Source: three-view drawing plus pictorial views. Frame: mm from the lowest corner of the part. A direction names the side the tool comes from. Coordinates: 2 decimals unless noted, no trailing zeros. Order: outer loops, then holes, each group sorted by start corner. A loop starts at its lowest first (then second) coordinate and runs counter-clockwise, first axis right, second up. Notation, with made-up numbers: M -14.5,86.25 L -3.5,86.25 A31 cw -3.5,123.25 Z; hole C -1,-7.5 d7. An arc over 180 degrees is marked long. One line per question, with ' | ' between items.
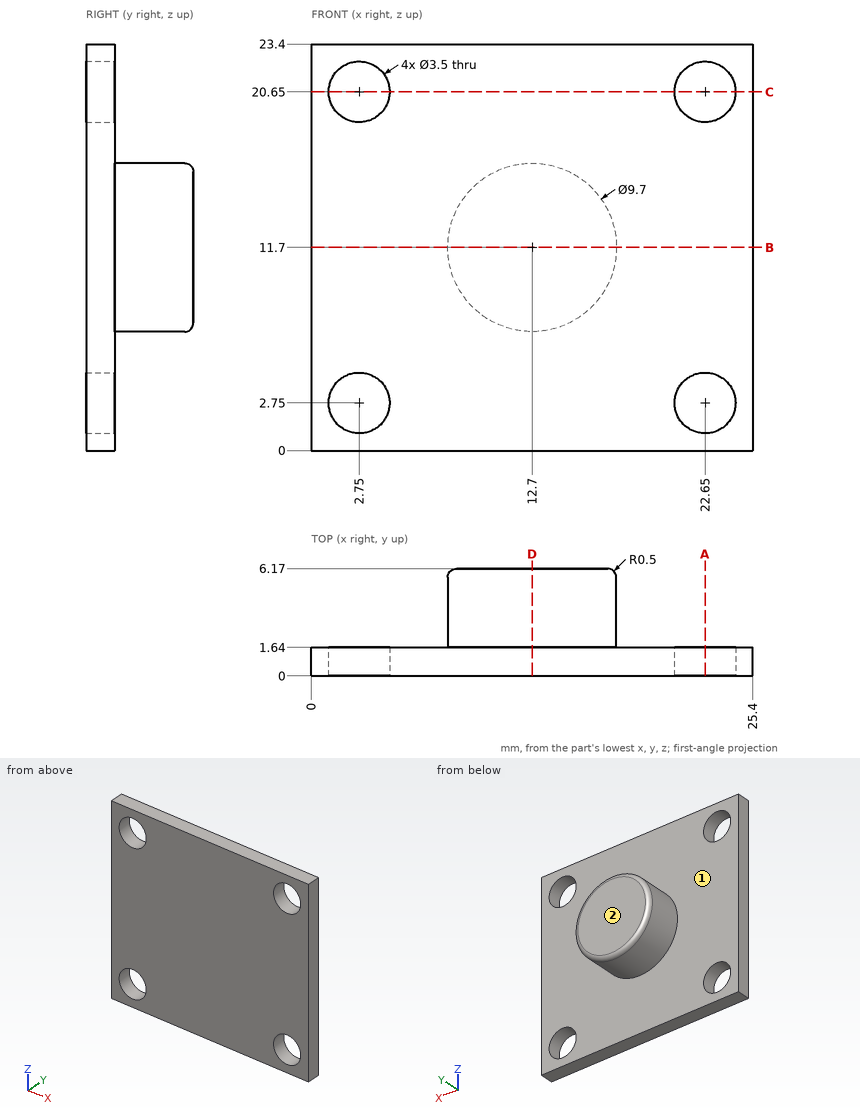
1. Section C-C, the plane z = 20.65. Output: boundary loops of the cut face in (x, y).
Response values:
outline: M 0,0 L 1,0 L 1,1.64 L 0,1.64 Z; M 4.5,0 L 20.9,0 L 20.9,1.64 L 4.5,1.64 Z; M 24.4,0 L 25.4,0 L 25.4,1.64 L 24.4,1.64 Z
2. Section D-D, the plane x = 12.7. Output: boundary loops of the cut face in (y, z), and give its area (3 significant figures).
Response values:
outline: M 0,0 L 1.64,0 L 1.64,6.85 L 5.67,6.85 A0.5 ccw 6.17,7.35 L 6.17,16.05 A0.5 ccw 5.67,16.55 L 1.64,16.55 L 1.64,23.4 L 0,23.4 Z | area: 82.2 mm^2
3. Access query for the marked faces 1 and 2. Directions: +Z, -Z, +X, -X, +Y, -Y. A direction counts if a zero-diameter tool reaches every point of the face in a straight line with its end or side. Return the directions, or none.
Response values:
face 1: +Y | face 2: +Z, -Z, +X, -X, +Y
4. Pin query (flat end, axial travel): P1, Ø5.5, axis at x = 2.75, z = 2.75, coming from the +Y side; P2, Ø1, axis at y = 4, z = 8, coming from the -X side. Return the tip coordinate at first contact, or that it passes through.
Response values:
P1: stops at y = 1.64 | P2: stops at x = 9.06
5. Section A-A, the plane x = 22.65. Output: boundary loops of the cut face in (y, z), and give its area (3 significant figures).
Response values:
outline: M 0,0 L 1.64,0 L 1.64,1 L 0,1 Z; M 0,4.5 L 1.64,4.5 L 1.64,18.9 L 0,18.9 Z; M 0,22.4 L 1.64,22.4 L 1.64,23.4 L 0,23.4 Z | area: 26.9 mm^2
6. Material intervals for line 1 (X direction, y = 1.35, z = 20.65); line 2 (Z direction, x = 22.65, y = 0.7); line 3 (Y direction, x = 6, z = 2.75), sorted ascending. Write a range as [from, to].
Response values:
line 1: x = [0, 1], [4.5, 20.9], [24.4, 25.4] | line 2: z = [0, 1], [4.5, 18.9], [22.4, 23.4] | line 3: y = [0, 1.64]
7. Section B-B, the plane z = 11.7. Output: boundary loops of the cut face in (x, y).
Response values:
outline: M 0,0 L 25.4,0 L 25.4,1.64 L 17.55,1.64 L 17.55,5.67 A0.5 ccw 17.05,6.17 L 8.35,6.17 A0.5 ccw 7.85,5.67 L 7.85,1.64 L 0,1.64 Z
